```python
from build123d import *

# Parameters (mm, degrees)
BOSS_EXTRUDE1_DEPTH = 2.8956
SKETCH2_R           = 1.5875
CUT_EXTRUDE1_DEPTH  = 2.8956
CHAMFER3_SIZE       = 0.254
CHAMFER4_SIZE       = 0.254


with BuildPart() as part:
    # Sketch1 → Boss-Extrude1 (new body)
    with BuildSketch(Plane(origin=(0, 0, 0), x_dir=(1, 0, 0), z_dir=(0, 1, 0))):
        Polygon((0, -4.575385413), (3.9624, -2.287692707), (3.9624, 2.287692707), (0, 4.575385413), (-3.9624, 2.287692707), (-3.9624, -2.287692707), align=None)
    extrude(amount=BOSS_EXTRUDE1_DEPTH)

    # Sketch2 → Cut-Extrude1 (cut)
    with BuildSketch(Plane(origin=(0, 2.8956, 0), x_dir=(1, 0, 0), z_dir=(0, 1, 0))):
        Circle(SKETCH2_R)
    extrude(amount=-CUT_EXTRUDE1_DEPTH, mode=Mode.SUBTRACT)

    # Chamfer3
    chamfer3_edges = [part.edges().sort_by_distance(p)[0] for p in [
        (-1.5875, 2.8956, 0),
    ]]
    chamfer(chamfer3_edges, length=CHAMFER3_SIZE)

    # Chamfer4
    chamfer4_edges = [part.edges().sort_by_distance(p)[0] for p in [
        (-1.5875, 0, 0),
    ]]
    chamfer(chamfer4_edges, length=CHAMFER4_SIZE)


solid = part.part
```
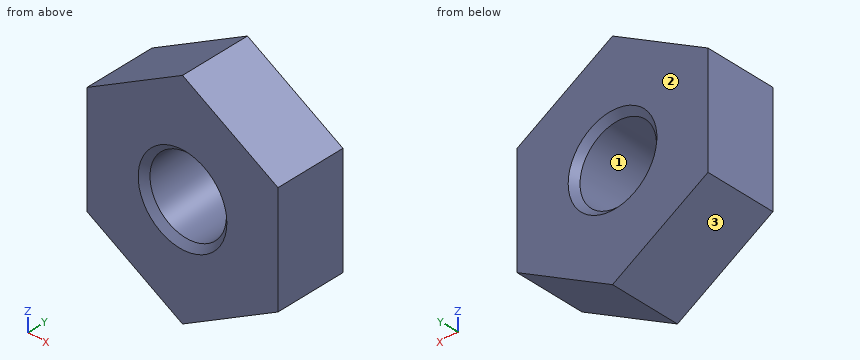
The model under review builds one solid part; all positions refer to its coordinate system, in mm. Face numbers are marked on the shaded views. Round coordinates to 2 decimals unless told otherwise and drop trailing zeros. Loops run counter-clockwise (first coordinate to the right, second up) from the corner with the lowest first, then second, coordinate; pieces in that order, holes last. Notation, with made-up numbers: M 78.5,37.5 L 109.5,37.5 A19 ccw 109.5,44.5 Z; hole C -24.75,45 d1. An arc over 180 degrees is marked long. Write item = value, one per line.
Item 1: Take a section at C-C on x = -2.25. Write out the cut boundary in (y, z).
Return value:
outline = M 0,-3.28 L 2.9,-3.28 L 2.9,3.28 L 0,3.28 Z
Item 2: Take a section at B-B on z = 0. Write out the cut boundary in (x, y).
Return value:
outline = M -3.96,0 L -1.84,0 L -1.59,0.25 L -1.59,2.64 L -1.84,2.9 L -3.96,2.9 Z; M 1.59,0.25 L 1.84,0 L 3.96,0 L 3.96,2.9 L 1.84,2.9 L 1.59,2.64 Z
Item 3: Take a section at A-A on y = 2.15. Write out the cut boundary in (x, z) (1 decimal), then the cut area to 3 significant figures.
Return value:
outline = M -4,-2.3 L 0,-4.6 L 4,-2.3 L 4,2.3 L 0,4.6 L -4,2.3 Z; hole C 0,0 d3.2
area = 46.5 mm2
Item 4: For line 1 (X direction, y = 2.15, z = 0); line 2 (X direction, y = 1.65, z = 1.25); line 3 (Z direction, x = 0.75, y = 0.3), list the stretches that pass through material, from the lowest coordinate up. Write a range as [from, to].
Return value:
line_1 = [-3.96, -1.59], [1.59, 3.96]
line_2 = [-3.96, -0.98], [0.98, 3.96]
line_3 = [-4.14, -1.4], [1.4, 4.14]
Item 5: Take a section at D-D on z = -2.75. Write out the cut boundary in (x, y), then the cut area to 3 significant figures.
Return value:
outline = M -3.16,0 L 3.16,0 L 3.16,2.9 L -3.16,2.9 Z
area = 18.3 mm2
Item 6: The part is to be moulded in two halves that separate along X. For the marked faces 1, 2 and 3, say which applies: released by +X, released by -X, zero draft, split by the parting line, or undercut.
Return value:
face_1 = undercut
face_2 = zero draft
face_3 = released by -X
